Build history of the part. All positions in model axes, mm. A direction names the side the tool comes from. Coordinates: 2 decimals unless noted, no trailing zeros. Order: outer loops, then holes, each group sorted by start corner. A loop starts at its lowest first (then second) coordinate and runs counter-clockwise, first axis right, second up. Notation, with made-up numbers: (38, 48) - (79, 48) arc R27 ccw to (79, 65) - close; hole circle Ø5 at (82, 40). An arc over 180 degrees is marked (long way). Return JSON: item names as keys, results as strings.
from build123d import *

# Parameters (mm, degrees)
SKETCH1_W           = 6
SKETCH1_H           = 5
BOSS_EXTRUDE1_DEPTH = 6
CUT_EXTRUDE1_DEPTH  = 2.5
CUT_EXTRUDE2_DEPTH  = 2.5


with BuildPart() as part:
    # Sketch1 → Boss-Extrude1 (new body)
    with BuildSketch(Plane(origin=(0, 0, 0), x_dir=(1, 0, 0), z_dir=(0, 1, 0))):
        Rectangle(SKETCH1_W, SKETCH1_H)
    extrude(amount=BOSS_EXTRUDE1_DEPTH)

    # Sketch2 → Cut-Extrude1 (cut)
    with BuildSketch(Plane(origin=(0, 6, 0), x_dir=(1, 0, 0), z_dir=(0, 1, 0))):
        Polygon((3, -1), (0, -1), (0, 1), (-3, 1), (-3, -2.5), (3, -2.5), align=None)
    extrude(amount=-CUT_EXTRUDE1_DEPTH, mode=Mode.SUBTRACT)

    # Sketch3 → Cut-Extrude2 (cut)
    with BuildSketch(Plane.XZ):
        Polygon((3, 1), (0, 1), (0, -1), (-3, -1), (-3, 2.5), (3, 2.5), align=None)
    extrude(amount=-CUT_EXTRUDE2_DEPTH, mode=Mode.SUBTRACT)


solid = part.part
1. Cut at C-C on y = 5. Give the cut face in (x, z).
Check values:
{"outline": "(-3, -2.5) - (3, -2.5) - (3, 1) - (0, 1) - (0, -1) - (-3, -1) - close"}
2. Drop flat-ended pins along their axis: pin 1 (0.8 mm diameter, centred on x = 1, y = 1, fed in from +Z); pin 2 (2 mm diameter, centred on y = 5, z = 0.5, fed in from -X); pin 3 (1.2 mm diameter, centred on x = -1, y = 1.5, fed in from +Z). Give the stop position or say it passes through.
Check values:
{"pin 1": "z = 1", "pin 2": "x = 0", "pin 3": "z = -1"}
3. Probe L1, parallel to Y at x = 0.55, z = 1.5; L2, parallel to X at y = 4.95, z = -0.2; L3, parallel to Z at x = 2.3, y = 5.5. List the from-to ranges inside material, lowest first.
Check values:
{"L1": "2.5 to 3.5", "L2": "0 to 3", "L3": "-2.5 to 1"}
4. Tool access for faces 1 (the flat face through (3, 3, -1)), 2 (the flat face through (2, 5, 1)), 3 (the flat face through (0, 5, 0)), 4 (the flat face through (2, 1, 1)), 5 (the flat face through (-1, 1, -1)): list every direction of +Z, -Z, +X, -X, +Y, -Y with a clear straight run to the whole face (end or side of a thin tool).
Check values:
{"face 1": "+Z, -Z, +X, +Y, -Y", "face 2": "+Z, +X, -X, +Y", "face 3": "+Z, -X, +Y", "face 4": "+Z, +X, -X, -Y", "face 5": "+Z, -X, -Y"}
5. Cut at D-D on z = 1.55. Give the cut face in (x, y), plus the area to 3 significant figures.
Check values:
{"outline": "(-3, 2.5) - (3, 2.5) - (3, 3.5) - (-3, 3.5) - close", "area": "6.00 mm²"}
6. Cut at B-B on x = 0.8. Give the cut face in (y, z), plus the area to 3 significant figures.
Check values:
{"outline": "(0, -2.5) - (6, -2.5) - (6, 1) - (3.5, 1) - (3.5, 2.5) - (2.5, 2.5) - (2.5, 1) - (0, 1) - close", "area": "22.5 mm²"}
7. Cut at A-A on z = 0.7. Give the cut face in (x, y).
Check values:
{"outline": "(-3, 2.5) - (0, 2.5) - (0, 0) - (3, 0) - (3, 6) - (0, 6) - (0, 3.5) - (-3, 3.5) - close"}
